```python
from build123d import *

# Parameters (mm, degrees)
SKETCH_1_R          = 9.5
SKETCH_1_R_2        = 5
EXTRUDE_1_DEPTH     = 5
EXTRUDE_START       = -1.5
SKETCH_2_R          = 11
SKETCH_2_R_2        = 9.5
EXTRUDE_2_DEPTH     = 1.5
SKETCH_3_R          = 8
SKETCH_3_R_2        = 6
CUT_EXTRUDE_1_DEPTH = 1
CUT_EXTRUDE_START   = -1
SKETCH_4_R          = 8
SKETCH_4_R_2        = 6
CUT_EXTRUDE_2_DEPTH = 1
CHAMFER_1_SIZE      = 0.3


with BuildPart() as part:
    # Эскиз1 → Бобышка-Вытянуть1 (new body)
    with BuildSketch(Plane.XY):
        Circle(SKETCH_1_R)
        Circle(SKETCH_1_R_2, mode=Mode.SUBTRACT)
    extrude(amount=EXTRUDE_1_DEPTH)

    # Эскиз2 → Бобышка-Вытянуть2 (add)
    with BuildSketch(Plane.XY.offset(5).offset(EXTRUDE_START)):
        Circle(SKETCH_2_R)
        Circle(SKETCH_2_R_2, mode=Mode.SUBTRACT)
    extrude(amount=EXTRUDE_2_DEPTH)

    # Эскиз3 → Вырез-Вытянуть1 (cut)
    with BuildSketch(Plane(origin=(0, 0, 0), x_dir=(-1, 0, 0), z_dir=(0, 0, -1))):
        Circle(SKETCH_3_R)
        Circle(SKETCH_3_R_2, mode=Mode.SUBTRACT)
    extrude(amount=-CUT_EXTRUDE_1_DEPTH, mode=Mode.SUBTRACT)

    # Эскиз4 → Вырез-Вытянуть2 (cut)
    with BuildSketch(Plane.XY.offset(5).offset(CUT_EXTRUDE_START)):
        with Locations(Location((0, 0, 0), (0, 0, 180))):
            Circle(SKETCH_4_R)
        with Locations(Location((0, 0, 0), (0, 0, 180))):
            Circle(SKETCH_4_R_2, mode=Mode.SUBTRACT)
    extrude(amount=CUT_EXTRUDE_2_DEPTH, mode=Mode.SUBTRACT)

    # Фаска1
    chamfer_1_edges = [part.edges().sort_by_distance(p)[0] for p in [
        (-11, 0, 3.5),
        (-11, 0, 5),
        (8, 0, 0),
        (6, 0, 0),
        (-9.5, 0, 0),
        (8, 0, 5),
        (6, 0, 5),
        (-5, 0, 0),
        (-5, 0, 5),
    ]]
    chamfer(chamfer_1_edges, length=CHAMFER_1_SIZE)


solid = part.part
```
Check sheet for the modelled part. Datum: model origin and axes. Units: mm. A direction names the side the tool comes from. Round coordinates to 2 decimals unless told otherwise and drop trailing zeros. Loops run counter-clockwise (first coordinate to the right, second up) from the corner with the lowest first, then second, coordinate; pieces in that order, holes last. Notation, with made-up numbers: (-14.5, 16.25) -> (28.5, 16.25) arc R16 ccw to (28.5, 31.25) -> close; hole circle Ø6 at (-11, 45.25). An arc over 180 degrees is marked (long way). Write item = value, one per line. Start each with the question number.
1) Sectioned sample at A-A, the plane z = 0.65. Record the cut outline in (x, y).
2) Thickness scan on probe 1 along Y at (x, z) = (0, 0.85); probe 2 along Y at (x, z) = (0, 4.25); probe 3 along Y at (x, z) = (0, 2.85). Record the ranges inside material, lowest first.
3) Sectioned sample at B-B, the plane z = 2.4. Record the cut outline in (x, y), plus the area to 3 significant figures.
4) Set-up check for faces 1 (the flat face through (2, 6, 1)), 2 (the cylindrical face through (1.73, 7.81, 4.35)), 3 (the flat face through (-5, 7, 0)): record each of +Z, -Z, +X, -X, +Y, -Y from which the full face is reachable in a straight line by a thin tool's end or side.
5) Gauge pin test, flat ends, axial feed: pin 1 Ø3 at (x, y) = (-1, -2) entering from -Z; pin 2 Ø2 at (x, z) = (-5.5, 4) entering from -Y; pin 3 Ø2 at (x, z) = (8.5, 4.5) entering from +Y. Record the tip position at first contact, or that the pin passes through.
6) Release check for a two-part mould opening along X. For faces 4 (the cylindrical face through (4.38, -8.43, 1.88)), 5 (the flat face through (0, 10, 3.5)), 6 (the cylindrical face through (-5.723, -1.802, 4.345)) record: released by +X, released by -X, zero draft, split by the parting line, or undercut.
Results are:
q1.outline = circle Ø19 at (0, 0); circle Ø12 at (0, 0); hole circle Ø16 at (0, 0); hole circle Ø10 at (0, 0)
q2.probe_1 = -9.5 to -8, -6 to -5, 5 to 6, 8 to 9.5
q2.probe_2 = -11 to -8, -6 to -5, 5 to 6, 8 to 11
q2.probe_3 = -9.5 to -5, 5 to 9.5
q3.outline = circle Ø19 at (0, 0); hole circle Ø10 at (0, 0)
q3.area = 205 mm^2
q4.face_1 = -Z
q4.face_2 = +Z
q4.face_3 = -Z, +X, -X, +Y, -Y
q5.pin_1 = through
q5.pin_2 = -10.04
q5.pin_3 = 8.05
q6.face_4 = split by the parting line
q6.face_5 = zero draft
q6.face_6 = undercut
